Read the model definition and answer for the solid it produces. Units are mm, in the model's axes. A direction names the side the tool comes from. Give positions to 0.01 mm unless a question says otherwise; leave off trailing zeros. Write item = value, one per line.
```python
from build123d import *

# Parameters (mm, degrees)
BOSS_EXTRUDE1_DEPTH = 81
SKETCH10_W          = 50
SKETCH10_H          = 4.1


with BuildPart() as part:
    # Sketch1 → Boss-Extrude1 (new body)
    with BuildSketch(Plane(origin=(0, 0, 0), x_dir=(0, 0, -1), z_dir=(1, 0, 0))):
        with BuildLine():
            Line((-15, -32), (-5, -32))
            Line((-5, -32), (-4.2, -31.2))
            Line((-4.2, -31.2), (5.866666667, -31.2))
            Line((5.866666667, -31.2), (6.666666667, -32))
            Line((6.666666667, -32), (15, -32))
            Line((15, -32), (15, -22.434782609))
            Line((15, -22.434782609), (14.5, -22.434782609))
            Line((14.5, -22.434782609), (14.5, -19.633333333))
            Line((14.5, -19.633333333), (12.5, -17.5))
            Line((12.5, -17.5), (15, -14.833333333))
            Line((15, -14.833333333), (15, -9.714205686))
            Line((15, -9.714205686), (13.235294118, -7.611111111))
            Line((13.235294118, -7.611111111), (13.235294118, -6.044444444))
            ThreePointArc((13.235294118, -6.044444444), (12.988775356, -6.313226652), (12.706722689, -6.544444444))
            Line((12.706722689, -6.544444444), (9.735294118, -6.544444444))
            ThreePointArc((9.735294118, -6.544444444), (8.674633946, -6.105104616), (8.235294118, -5.044444444))
            Line((8.235294118, -5.044444444), (8.235294118, -3.844444444))
            ThreePointArc((8.235294118, -3.844444444), (8.674633946, -2.783784273), (9.735294118, -2.344444444))
            Line((9.735294118, -2.344444444), (12.706722689, -2.344444444))
            ThreePointArc((12.706722689, -2.344444444), (12.988775356, -2.575662237), (13.235294118, -2.844444444))
            Line((13.235294118, -2.844444444), (13.235294118, 2.844444444))
            ThreePointArc((13.235294118, 2.844444444), (12.988775356, 2.575662237), (12.706722689, 2.344444444))
            Line((12.706722689, 2.344444444), (9.735294118, 2.344444444))
            ThreePointArc((9.735294118, 2.344444444), (8.674633946, 2.783784273), (8.235294118, 3.844444444))
            Line((8.235294118, 3.844444444), (8.235294118, 5.044444444))
            ThreePointArc((8.235294118, 5.044444444), (8.674633946, 6.105104616), (9.735294118, 6.544444444))
            Line((9.735294118, 6.544444444), (12.706722689, 6.544444444))
            ThreePointArc((12.706722689, 6.544444444), (12.988775356, 6.313226652), (13.235294118, 6.044444444))
            Line((13.235294118, 6.044444444), (13.235294118, 7.611111111))
            Line((13.235294118, 7.611111111), (15, 9.714205686))
            Line((15, 9.714205686), (15, 14.833333333))
            Line((15, 14.833333333), (12.5, 17.5))
            Line((12.5, 17.5), (14.5, 19.633333333))
            Line((14.5, 19.633333333), (14.5, 22.434782609))
            Line((14.5, 22.434782609), (15, 22.434782609))
            Line((15, 22.434782609), (15, 32))
            Line((15, 32), (6.666666667, 32))
            Line((6.666666667, 32), (5.866666667, 31.2))
            Line((5.866666667, 31.2), (-4.2, 31.2))
            Line((-4.2, 31.2), (-5, 32))
            Line((-5, 32), (-15, 32))
            Line((-15, 32), (-15, 15))
            Line((-15, 15), (-13.2679, 12))
            Line((-13.2679, 12), (-15, 9))
            Line((-15, 9), (-15, 7))
            Line((-15, 7), (-14.7, 6.7))
            Line((-14.7, 6.7), (-14.7, 5.42))
            ThreePointArc((-14.7, 5.42), (-14.453481239, 5.688782207), (-14.171428571, 5.92))
            Line((-14.171428571, 5.92), (-11.2, 5.92))
            ThreePointArc((-11.2, 5.92), (-10.139339828, 5.480660172), (-9.7, 4.42))
            Line((-9.7, 4.42), (-9.7, 3.22))
            ThreePointArc((-9.7, 3.22), (-10.139339828, 2.159339828), (-11.2, 1.72))
            Line((-11.2, 1.72), (-14.171428571, 1.72))
            ThreePointArc((-14.171428571, 1.72), (-14.453481239, 1.951217793), (-14.7, 2.22))
            Line((-14.7, 2.22), (-14.7, -3.468888889))
            ThreePointArc((-14.7, -3.468888889), (-14.453481239, -3.200106681), (-14.171428571, -2.968888889))
            Line((-14.171428571, -2.968888889), (-11.2, -2.968888889))
            ThreePointArc((-11.2, -2.968888889), (-10.139339828, -3.408228717), (-9.7, -4.468888889))
            Line((-9.7, -4.468888889), (-9.7, -5.668888889))
            ThreePointArc((-9.7, -5.668888889), (-10.139339828, -6.729549061), (-11.2, -7.168888889))
            Line((-11.2, -7.168888889), (-14.171428571, -7.168888889))
            ThreePointArc((-14.171428571, -7.168888889), (-14.453481239, -6.937671096), (-14.7, -6.668888889))
            Line((-14.7, -6.668888889), (-14.7, -6.7))
            Line((-14.7, -6.7), (-15, -7))
            Line((-15, -7), (-15, -9))
            Line((-15, -9), (-13.2679, -12))
            Line((-13.2679, -12), (-15, -15))
            Line((-15, -15), (-15, -32))
        make_face()
    extrude(amount=BOSS_EXTRUDE1_DEPTH)

    # Sketch2 → Cut-Revolve1 (revolve, cut)
    with BuildSketch(Plane.XY):
        Polygon((0, 23), (0, 27.6), (0.5, 27.1), (80.5, 27.1), (81, 27.6), (81, 23), align=None)
    revolve(axis=Axis((81, 23, 0), (-1, 0, 0)), mode=Mode.SUBTRACT)

    # Sketch3 → Cut-Revolve2 (revolve, cut)
    with BuildSketch(Plane.XY):
        Polygon((0, -23), (0, -18.4), (0.5, -18.9), (80.5, -18.9), (81, -18.4), (81, -23), align=None)
    revolve(axis=Axis((81, -23, 0), (-1, 0, 0)), mode=Mode.SUBTRACT)

    # Sketch4 → Cut-Revolve3 (revolve, cut)
    with BuildSketch(Plane(origin=(0, 27, 0), x_dir=(-1, 0, 0), z_dir=(0, 1, 0))):
        Polygon((-11, -15), (-13.5, -15), (-13.067, -14.567), (-13.067, -7.093383006), (-11, -5.9), align=None)
    revolve(axis=Axis((11, 27, -5.9), (0, 0, -1)), mode=Mode.SUBTRACT)

    # Sketch5 → Cut-Revolve4 (revolve, cut)
    with BuildSketch(Plane(origin=(0, 27, 0), x_dir=(-1, 0, 0), z_dir=(0, 1, 0))):
        Polygon((-68, -15), (-70.5, -15), (-70.067, -14.567), (-70.067, -7.093383006), (-68, -5.9), align=None)
    revolve(axis=Axis((68, 27, -5.9), (0, 0, -1)), mode=Mode.SUBTRACT)

    # Sketch6 → Cut-Revolve5 (revolve, cut)
    with BuildSketch(Plane(origin=(0, -27, 0), x_dir=(-1, 0, 0), z_dir=(0, 1, 0))):
        Polygon((-11, -15), (-13.5, -15), (-13.067, -14.567), (-13.067, -7.093383006), (-11, -5.9), align=None)
    revolve(axis=Axis((11, -27, -5.9), (0, 0, -1)), mode=Mode.SUBTRACT)

    # Sketch7 → Cut-Revolve6 (revolve, cut)
    with BuildSketch(Plane(origin=(0, -27, 0), x_dir=(-1, 0, 0), z_dir=(0, 1, 0))):
        Polygon((-68, -15), (-70.5, -15), (-70.067, -14.567), (-70.067, -7.093383006), (-68, -5.9), align=None)
    revolve(axis=Axis((68, -27, -5.9), (0, 0, -1)), mode=Mode.SUBTRACT)

    # Sketch8 → Cut-Revolve7 (revolve, cut)
    with BuildSketch(Plane(origin=(0, -23, 0), x_dir=(-1, 0, 0), z_dir=(0, 1, 0))):
        Polygon((-11, 9.25), (-13.067, 9.25), (-13.067, 14.567), (-13.5, 15), (-11, 15), align=None)
    revolve(axis=Axis((11, -23, 15), (0, 0, -1)), mode=Mode.SUBTRACT)

    # Sketch9 → Cut-Revolve8 (revolve, cut)
    with BuildSketch(Plane(origin=(0, -23, 0), x_dir=(-1, 0, 0), z_dir=(0, 1, 0))):
        Polygon((-64, 9.25), (-66.067, 9.25), (-66.067, 14.567), (-66.5, 15), (-64, 15), align=None)
    revolve(axis=Axis((64, -23, 15), (0, 0, -1)), mode=Mode.SUBTRACT)

    # Sketch10 → Cut-Revolve9 (revolve, cut)
    with BuildSketch(Plane(origin=(0, 0, 0), x_dir=(-1, 0, 0), z_dir=(0, 1, 0))):
        with Locations((-25, -2.05)):
            Rectangle(SKETCH10_W, SKETCH10_H)
    revolve(axis=Axis((50, 0, 0), (-1, 0, 0)), mode=Mode.SUBTRACT)

    # Sketch11 → Cut-Revolve10 (revolve, cut)
    with BuildSketch(Plane(origin=(11, 0, 0), x_dir=(0, 0, -1), z_dir=(1, 0, 0))):
        Polygon((-10, -26), (-7.933, -26), (-7.933, -31.567), (-7.5, -32), (-10, -32), align=None)
    revolve(axis=Axis((11, -32, 10), (0, 1, 0)), mode=Mode.SUBTRACT)

    # Sketch12 → Cut-Revolve11 (revolve, cut)
    with BuildSketch(Plane(origin=(64, 0, 0), x_dir=(0, 0, -1), z_dir=(1, 0, 0))):
        Polygon((-10, -26), (-7.933, -26), (-7.933, -31.567), (-7.5, -32), (-10, -32), align=None)
    revolve(axis=Axis((64, -32, 10), (0, 1, 0)), mode=Mode.SUBTRACT)

    # Sketch13 → Cut-Revolve12 (revolve, cut)
    with BuildSketch(Plane.XY):
        Polygon((71.556624327, 0), (73, 2.5), (81, 2.5), (81, 0), align=None)
    revolve(axis=Axis((81, 0, 0), (-1, 0, 0)), mode=Mode.SUBTRACT)

    # Sketch14 → Cut-Revolve13 (revolve, cut)
    with BuildSketch(Plane.XY.offset(-11)):
        Polygon((66.606616994, 21), (67.8, 23.067), (80.567, 23.067), (81, 23.5), (81, 21), align=None)
    revolve(axis=Axis((81, 21, -11), (-1, 0, 0)), mode=Mode.SUBTRACT)

    # Sketch15 → Cut-Revolve14 (revolve, cut)
    with BuildSketch(Plane.XY.offset(-11)):
        Polygon((66.606616994, -21), (67.8, -18.933), (80.567, -18.933), (81, -18.5), (81, -21), align=None)
    revolve(axis=Axis((81, -21, -11), (-1, 0, 0)), mode=Mode.SUBTRACT)

    # Sketch16 → Cut-Revolve15 (revolve, cut)
    with BuildSketch(Plane.XY.offset(11)):
        Polygon((66.606616994, 21), (67.8, 23.067), (80.567, 23.067), (81, 23.5), (81, 21), align=None)
    revolve(axis=Axis((81, 21, 11), (-1, 0, 0)), mode=Mode.SUBTRACT)

    # Sketch17 → Cut-Revolve16 (revolve, cut)
    with BuildSketch(Plane.XY.offset(11)):
        Polygon((66.606616994, -21), (67.8, -18.933), (80.567, -18.933), (81, -18.5), (81, -21), align=None)
    revolve(axis=Axis((81, -21, 11), (-1, 0, 0)), mode=Mode.SUBTRACT)

    # Sketch18 → Cut-Revolve17 (revolve, cut)
    with BuildSketch(Plane(origin=(5, 0, 0), x_dir=(0, 0, -1), z_dir=(1, 0, 0))):
        Polygon((-15, 12), (-15, 16), (-10.5, 16), (-10.5, 14.15), (4.393782217, 14.15), (4.393782217, 14.067), (14.567, 14.067), (15, 14.5), (15, 12), align=None)
    revolve(axis=Axis((5, 12, -15), (0, 0, 1)), mode=Mode.SUBTRACT)

    # Sketch19 → Cut-Revolve18 (revolve, cut)
    with BuildSketch(Plane(origin=(5, 0, 0), x_dir=(0, 0, -1), z_dir=(1, 0, 0))):
        Polygon((-15, -12), (-15, -8), (-10.5, -8), (-10.5, -9.85), (4.393782217, -9.85), (4.393782217, -9.933), (14.567, -9.933), (15, -9.5), (15, -12), align=None)
    revolve(axis=Axis((5, -12, -15), (0, 0, 1)), mode=Mode.SUBTRACT)

    # Sketch20 → Cut-Revolve19 (revolve, cut)
    with BuildSketch(Plane(origin=(59, 0, 0), x_dir=(0, 0, -1), z_dir=(1, 0, 0))):
        Polygon((-15, -12), (-15, -8), (-10.5, -8), (-10.5, -9.85), (4.393782217, -9.85), (4.393782217, -9.933), (14.567, -9.933), (15, -9.5), (15, -12), align=None)
    revolve(axis=Axis((59, -12, -15), (0, 0, 1)), mode=Mode.SUBTRACT)

    # Sketch21 → Cut-Revolve20 (revolve, cut)
    with BuildSketch(Plane(origin=(59, 0, 0), x_dir=(0, 0, -1), z_dir=(1, 0, 0))):
        Polygon((-15, 12), (-15, 16), (-10.5, 16), (-10.5, 14.15), (4.393782217, 14.15), (4.393782217, 14.067), (14.567, 14.067), (15, 14.5), (15, 12), align=None)
    revolve(axis=Axis((59, 12, -15), (0, 0, 1)), mode=Mode.SUBTRACT)


solid = part.part
```
1) The mould has two halves that part along X. Classify faces 1 (the face through (40, -32, 10)), 2 (the face through (9.48, -24.4, 11.95)): pulls with the +X half, pulls with the -X half, needs draft (parallel to the pull), parting line crosses it, or undercut.
Output:
face_1 = needs draft
face_2 = undercut
2) Find the intervals of material crossed by probe 1 along Y at (x, z) = (76.5, -11); probe 2 along X at (y, z) = (-12, -5.5); probe 3 along Y at (x, z) = (59, 12.1), in increasing order.
Output:
probe_1 = -32 to -23.07, -18.93 to -6.54, -2.34 to 2.34, 6.54 to 18.93, 23.07 to 32
probe_2 = 0 to 2.93, 7.07 to 56.93, 61.07 to 81
probe_3 = -32 to -16, -8 to -7.17, -2.97 to 1.72, 5.92 to 8, 16 to 32
3) Each of these flat-tipped pins is pushed along its axis until it touches: P1, Ø0.6, axis at x = 23.5, y = 4.5, coming from the -Z side; P2, Ø2.5, axis at y = -1, z = -0.5, coming from the -X side; P3, Ø3.5, axis at x = 59, y = 12, coming from the -Z side; P4, Ø1.3, axis at x = 23.5, y = -6.5, coming from the -Z side. Where does it stop, or does it pass through?
Output:
P1 = -8.24
P2 = 50
P3 = through
P4 = -13.24
4) A cutting plane is placed at A-A on x = 59. Give the number of separate pieces and of enclosed holes in the cut face, then the cut area to 3 significant figures.
Output:
separate_pieces = 3
enclosed_holes = 2
area = 1,380 mm²
5) A tool of negligible diameter and unlimited length cuts with its end or side. For faces 3 (the face through (31.659, -13.479, 14.122)), 4 (the face through (40, -21, -14.5)), 5 (the face through (24.65, -4.065, 0.534)), 6 (the face through (61.95, -28.82, 10.27)), 7 (the face through (8.905, -12.867, 12.719)), from which of +Z, -Z, +X, -X, +Y, -Y can it reach the whole face along a straight path? Write none if from no direction.
Output:
face_3 = +Z, +X, -X
face_4 = -Z, +X, -X
face_5 = -X
face_6 = -Y
face_7 = +Z
